The model under review builds one solid part; all positions refer to its coordinate system, in mm. A direction names the side the tool comes from. Round coordinates to 2 decimals unless told otherwise and drop trailing zeros. Write each loop counter-clockwise with the first axis right and the second up, starting at its lowest first coordinate (ties: lowest second). Pieces come first, ordered by that corner, then holes.
Item 1: Add section C-C (x = -53.5). Give the boundary of the cut face in (y, z).
Item 2: Clearance check with a flat-ended pin moving along its axis: pin 1 Ø5 at (x, y) = (-85.5, -42.5) entering from +Z. State where the tip first meets the part, or that it passes through.
Item 3: Machinability: for faces 1 (the face through (10, 0, 8)), 2 (the face through (-55, -28, 0)), which of the approach directions +Z, -Z, +X, -X, +Y, -Y give a long, thin tool a straight path to every point of the face, cutting with its end or side? Answer none if there is none.
Item 4: Add section B-B (z = 56). Give the boundary of the cut face in (x, y), plus the area to 3 significant figures.
Item 5: To check wall thickness, follow L1, parallel to Z at x = -25.5, y = -39; L2, parallel to X at y = -4.5, z = 50.5. State the ranges of each line that lie inside material, in increasing order.
Item 6: Add section A-A (y = -34.5). Give the boundary of the cut face in (x, z), plus the area to 3 significant figures.
```python
from build123d import *

# Parameters (mm, degrees)
F0_W     = 55.142552
F0_H     = 57.551987
F1_DEPTH = 55.372
F2_W     = 55.142552
F2_H     = 57.551987
F3_DEPTH = 55.372
F4_W     = 55.142552
F4_H     = 57.551987
F5_DEPTH = 55.372
F6_W     = 57.551987
F6_H     = 55.372
F7_DEPTH = 55.372
F8_W     = 57.551987
F8_H     = 55.372
F9_DEPTH = 55.372


with BuildPart() as f1:
    # F0 (on Top) → F1 (new body)
    with BuildSketch(Plane.XY):
        with Locations((27.571276, -28.775993)):
            Rectangle(F0_W, F0_H)
    extrude(amount=F1_DEPTH)

    # F2 (on face) → F3 (join)
    with BuildSketch(Plane.XY.offset(55.372)):
        with Locations((27.571276, -28.775993)):
            Rectangle(F2_W, F2_H)
    extrude(amount=F3_DEPTH)

    # F4 (on face) → F5 (join)
    with BuildSketch(Plane(origin=(0, 0, 0), x_dir=(1, 0, 0), z_dir=(0, 0, -1))):
        with Locations((27.571276, 28.775993)):
            Rectangle(F4_W, F4_H)
    extrude(amount=F5_DEPTH)

    # F6 (on face) → F7 (join)
    with BuildSketch(Plane(origin=(0, 0, 0), x_dir=(0, -1, 0), z_dir=(-1, 0, 0))):
        with Locations((28.775993, -27.686)):
            Rectangle(F6_W, F6_H)
    extrude(amount=F7_DEPTH)

    # F8 (on face) → F9 (join)
    with BuildSketch(Plane(origin=(-55.372, 0, 0), x_dir=(0, -1, 0), z_dir=(-1, 0, 0))):
        with Locations((28.775993, -27.686)):
            Rectangle(F8_W, F8_H)
    extrude(amount=F9_DEPTH)


solid = f1.part
```
Numbers:
1. outline: (-57.55, -55.37) - (0, -55.37) - (0, 0) - (-57.55, 0) - close
2. pin 1: stops at z = 0
3. face 1: +Z, -Z, +X, -X, +Y
3. face 2: +Z, -X, +Y, -Y
4. outline: (0, -57.55) - (55.14, -57.55) - (55.14, 0) - (0, 0) - close
4. area: 3,170 mm2
5. L1: z = -55.37 to 0
5. L2: x = 0 to 55.14
6. outline: (-110.74, -55.37) - (55.14, -55.37) - (55.14, 110.74) - (0, 110.74) - (0, 0) - (-110.74, 0) - close
6. area: 15,300 mm2
